Design review of the part built by this model. Coordinates are the model's own, in mm. A direction names the side the tool comes from. Round coordinates to 2 decimals unless told otherwise and drop trailing zeros. Write each loop counter-clockwise with the first axis right and the second up, starting at its lowest first coordinate (ties: lowest second). Pieces come first, ordered by that corner, then holes. Notation, with made-up numbers: (-3, 12) - (22, 12) arc R21 cw to (22, 40) - close; hole circle Ø8 at (70.5, 79.25). An arc over 180 degrees is marked (long way). Use one line per item in the form item = value.
```python
from build123d import *

# Parameters (mm, degrees)
SKETCH1_W                    = 694
SKETCH1_H                    = 33
BASE_FLANGE1_DEPTH           = 2
EDGE_FLANGE1_STRIP_W         = 12
EDGE_FLANGE1_STRIP_H         = 2
EDGE_FLANGE1_STRIP_CUT_DEPTH = 694
EDGE_FLANGE1_DEPTH           = 694
EDGE_FLANGE2_DEPTH           = 634


# Sheet-metal steps are written as plain solids
with BuildPart() as part:
    # Sketch1 → Base-Flange1 (new body)
    with BuildSketch(Plane.XY):
        Rectangle(SKETCH1_W, SKETCH1_H)
    extrude(amount=BASE_FLANGE1_DEPTH)

    # Edge-Flange1 strip (across the edge) → Edge-Flange1 strip cut (cut)
    with BuildSketch(Plane(origin=(347, -16.5, 0), x_dir=(0, 1, 0), z_dir=(-1, 0, 0))):
        with Locations((-2, -1)):
            Rectangle(EDGE_FLANGE1_STRIP_W, EDGE_FLANGE1_STRIP_H)
    extrude(amount=EDGE_FLANGE1_STRIP_CUT_DEPTH, mode=Mode.SUBTRACT)

    # Edge-Flange1 section (across the edge) → Edge-Flange1 (add)
    with BuildSketch(Plane(origin=(347, -16.5, 0), x_dir=(0, 1, 0), z_dir=(-1, 0, 0))):
        with BuildLine():
            Line((0, 2), (0, 25))
            Line((0, 25), (2, 25))
            Line((2, 25), (2, 2))
            ThreePointArc((2, 2), (2.585786438, 0.585786438), (4, 0))
            Line((4, 0), (4, -2))
            ThreePointArc((4, -2), (1.171572875, -0.828427125), (0, 2))
        make_face()
    extrude(amount=EDGE_FLANGE1_DEPTH)

    # Edge-Flange2 section (across the edge) → Edge-Flange2 (add)
    with BuildSketch(Plane(origin=(-317, 17.130597578, 0), x_dir=(0, -0.5735764363510416, -0.8191520442889949), z_dir=(1, 0, 0))):
        with BuildLine():
            Line((-2, 0.630597578), (-2, 11.369402422))
            Line((-2, 11.369402422), (0, 11.369402422))
            Line((0, 11.369402422), (0, 0.630597578))
            ThreePointArc((0, 0.630597578), (0.092566099, 0.029185979), (0.361695911, -0.516555295))
            Line((0.361695911, -0.516555295), (-1.276608177, -1.663708168))
            ThreePointArc((-1.276608177, -1.663708168), (-1.814867803, -0.57222562), (-2, 0.630597578))
        make_face()
    extrude(amount=EDGE_FLANGE2_DEPTH)


solid = part.part
```
Q1. We need section A-A on x = -242. Write out the cut boundary in (y, z).
Calculated:
outline = (-16.5, -25) - (-14.5, -25) - (-14.5, -2) arc R2 cw to (-12.5, 0) - (16.5, 0) arc R2 cw to (17.65, -0.36) - (26.44, -6.52) - (27.59, -4.88) - (18.79, 1.28) arc R4 ccw to (16.5, 2) - (-12.5, 2) arc R4 ccw to (-16.5, -2) - close
Q2. Draft analysis for pull direction Y (two halves, no side actions). For faces 3 (the flat face through (5, -16.5, -13)), 4 (the flat face through (-5, 2, 0)), 5 (the flat face through (347, -7.3, 0.4)), state which applies: released by +Y, released by -Y, zero draft, split by the parting line, or undercut.
Calculated:
face_3 = released by -Y
face_4 = undercut
face_5 = zero draft
Q3. For P1, Ø0.6, axis at x = 336, z = 1, coming from the +Y side; P2, Ø11.5, axis at x = 74, z = -15, coming from the +Y side; P3, Ø9.5, axis at y = 21.5, z = -2, coming from the -X side, all flat-tipped, find the tip position at first contact; note any pin that passes through.
Calculated:
P1 = 16.5
P2 = -14.5
P3 = -317
Q4. We need section B-B on z = -18.25. Write out the cut boundary in (x, y).
Calculated:
outline = (-347, -16.5) - (347, -16.5) - (347, -14.5) - (-347, -14.5) - close
Q5. Machinability: for faces 1 (the flat face through (5, -14.5, -14)), 2 (the flat face through (-347, -7.3, 0.4)), which of the approach directions +Z, -Z, +X, -X, +Y, -Y give a long, thin tool a straight path to every point of the face, cutting with its end or side? Answer none if there is none.
Calculated:
face_1 = -Z, +X, -X
face_2 = +Z, -Z, -X, +Y, -Y
Q6. To check wall thickness, follow line 1 along Z through (x, y) = (-140.5, -10); line 2 along Y through (x, z) = (191, -22); line 3 along Z through (x, y) = (78.5, -13.5). State the ranges of each line that lie inside material, in increasing order. Write a range as from..to.
Calculated:
line_1 = 0..2
line_2 = -16.5..-14.5
line_3 = -0.27..1.87
